Check sheet for the drawn part. Datum: minimum x, y, z corner. Units: mm. A direction names the side the tool comes from. Round coordinates to 2 decimals unless told otherwise and drop trailing zeros. Order: outer loops, then holes, each group sorted by start corner. A loop starts at its lowest first (then second) coordinate and runs counter-clockwise, first axis right, second up. Notation, with made-up numbers: (16, 38.25) -> (58, 38.25) arc R20 ccw to (58, 71.25) -> close; hole circle Ø7 at (29, -19). An arc over 180 degrees is marked (long way). Answer as a JSON object with one key per item and string values. Group by question number.
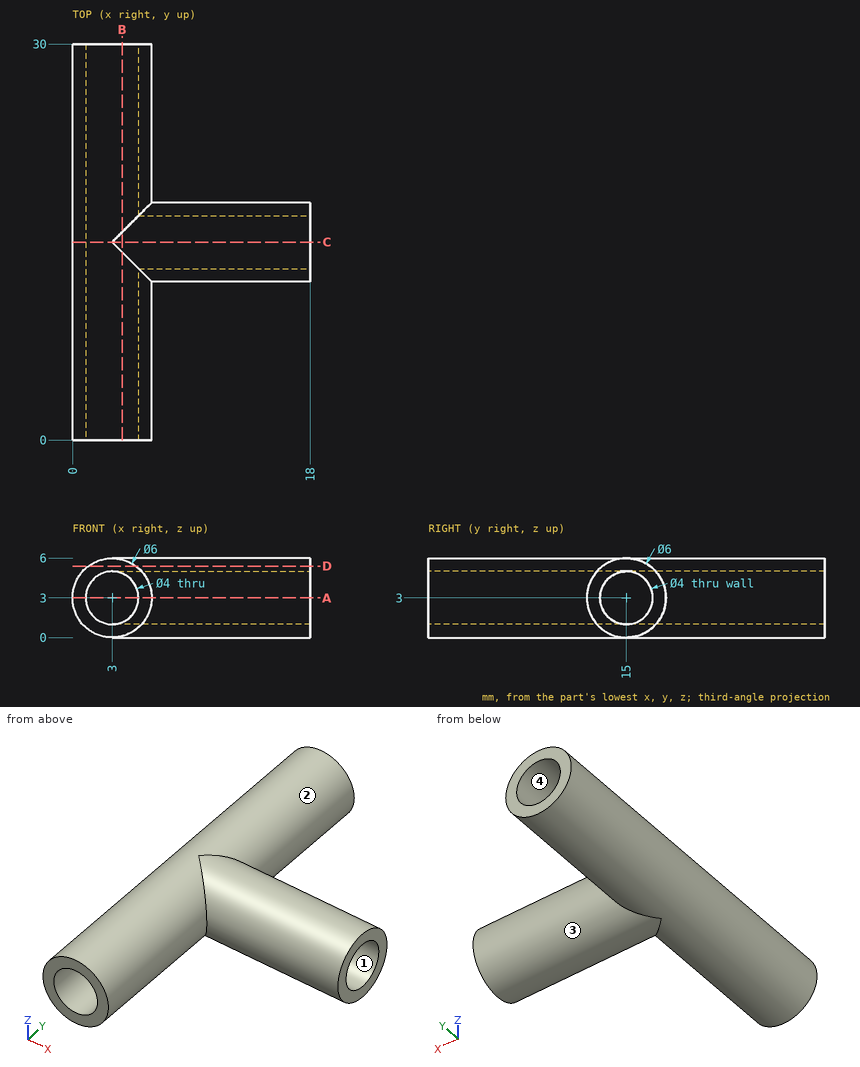
Item 1: Sectioned sample at B-B, the plane x = 3.75. Enter the section's corners in (y, z), then the cut area to 3 significant figures.
Item 2: Thickness scan on L1, parallel to X at y = 28, z = 2.85; L2, parallel to Z at x = 13, y = 15; L3, parallel to Y at x = 13.75, z = 2.9. Record the ranges inside material, lowest first.
Item 3: Sectioned sample at A-A, the plane z = 3. Enter the section's corners in (x, y).
Item 4: Sectioned sample at C-C, the plane y = 15. Enter the section's corners in (x, z).
Item 5: Sectioned sample at D-D, the plane z = 5.4. Enter the section's corners in (x, y), then the cut area to 3 significant figures.
Item 6: Depth check by flat-ended pin: pin 1 Ø1.5 at (y, z) = (14.5, 3) entering from +X; pin 2 Ø3 at (x, y) = (12.5, 13) entering from -Z. Enter the tip coordinate at first touch or a pass-through.
Item 7: Mould release check, pull along Z, two halves, no side actions. Record for the marked faces 3 and 4: pulls with the +Z half, pulls with the -Z half, needs draft (parallel to the pull), parting line crosses it, or undercut.
Item 8: Set-up check for the marked faces 1 and 2: record each of +Z, -Z, +X, -X, +Y, -Y from which the full face is reachable in a straight line by a thin tool's end or side.
Result:
{
 "1": {"outline": "(0, 0.1) -> (14.25, 0.1) arc R3 ccw to (15.75, 0.1) -> (30, 0.1) -> (30, 1.15) -> (15.75, 1.15) arc R2 cw to (14.25, 1.15) -> (0, 1.15) -> close; (0, 4.85) -> (14.25, 4.85) arc R2 cw to (15.75, 4.85) -> (30, 4.85) -> (30, 5.9) -> (15.75, 5.9) arc R3 ccw to (14.25, 5.9) -> (0, 5.9) -> close", "area": "62.9 mm2"},
 "2": {"L1": "x = 0 to 1.01, 4.99 to 6", "L2": "z = 0 to 1, 5 to 6", "L3": "y = 12 to 13, 17 to 18"},
 "3": {"outline": "(0, 0) -> (1, 0) -> (1, 30) -> (0, 30) -> close; (5, 0) -> (6, 0) -> (6, 12) -> (18, 12) -> (18, 13) -> (5, 13) -> close; (5, 17) -> (18, 17) -> (18, 18) -> (6, 18) -> (6, 30) -> (5, 30) -> close"},
 "4": {"outline": "(3, 0) -> (18, 0) -> (18, 1) -> (3, 1) arc R2 cw to (3, 5) -> (18, 5) -> (18, 6) -> (3, 6) arc R3 ccw to start"},
 "5": {"outline": "(1.2, 0) -> (4.8, 0) -> (4.8, 13.2) -> (18, 13.2) -> (18, 16.8) -> (4.8, 16.8) -> (4.8, 30) -> (1.2, 30) -> close", "area": "156 mm2"},
 "6": {"pin 1": "stops at x = 1.15", "pin 2": "stops at z = 0.04"},
 "7": {"face 3": "parting line crosses it", "face 4": "undercut"},
 "8": {"face 1": "+X", "face 2": "none"}
}
